Autodesk Inventor part; units mm, degrees
ref_plane "YZ Plane" through (0, 0, 0) normal (1, 0, 0) x (0, 1, 0)
ref_plane "XZ Plane" through (0, 0, 0) normal (0, 1, 0) x (-1, 0, 0)
ref_plane "XY Plane" through (0, 0, 0) normal (0, 0, 1) x (1, 0, 0)
sketch "Sketch1" plane through (0, 0, 0) normal (1, 0, 0) x (0, 1, 0)
  line L0 (109, 50) -> (-109, 50)
  line L1 (-109, 50) -> (-109, -50)
  line L2 (-109, -50) -> (109, -50)
  line L3 (109, -50) -> (109, 50)
  line L4 (109, 50) -> (-109, -50) construction
  line L5 (-109, 50) -> (109, -50) construction
  point P0 (0, 0)
  dimension "d0" = 100
  dimension "d1" = 218
extrude "Extrusion1" add sketch "Sketch1" along normal mid plane 10
sketch "Sketch2" plane through (-5, -109, 50) normal (0, 0, 1) x (1, 0, 0)
  line L0 (0, 218) -> (10, 218)
  line L1 (6, 218) -> (6, 196)
  line L2 (6, 196) -> (0, 190)
  line L3 (0, 218) -> (0, 0)
  line L4 (6, 218) -> (0, 218)
  line L5 (0, 190) -> (0, 218)
  line L6 (0, 0) -> (10, 0)
  line L7 (6, 0) -> (6, 60)
  line L8 (6, 60) -> (0, 60)
  line L9 (6, 0) -> (0, 0)
  line L10 (0, 60) -> (0, 0)
  point P0 (5, 109)
  dimension "d5" = 4
  dimension "d6" = 22
  dimension "d7" = 135
  dimension "d8" = 60
  dimension "d10" = 4
extrude "Extrusion2" cut sketch "Sketch2" against normal through all
sketch "Sketch3" plane through (5, 0, 0) normal (1, 0, 0) x (0, 0, -1)
  circle A0 centre (-38, -73) radius 4
  circle A1 centre (-23, -73) radius 4
  circle A2 centre (-8, -73) radius 4
  circle A3 centre (-33, 99) radius 4
  circle A4 centre (-18, 99) radius 4
  circle A5 centre (-3, 99) radius 4
  line L0 (-50, 109) -> (-50, -109)
  line L1 (-33, 99) -> (-18, 99) construction
  line L2 (-18, 99) -> (-3, 99) construction
  line L3 (50, 109) -> (-50, 109)
  line L4 (-38, -73) -> (-23, -73) construction
  line L5 (-23, -73) -> (-8, -73) construction
  line L6 (-50, -109) -> (50, -109)
  circle A6 centre (-20, 69) radius 5
  circle A7 centre (-5, 69) radius 5
  circle A8 centre (10, 69) radius 4
  circle A9 centre (-20, 9) radius 5
  circle A10 centre (-5, 9) radius 5
  circle A11 centre (10, 9) radius 4
  line L7 (-20, 69) -> (10, 69) construction
  line L8 (-20, 9) -> (10, 9) construction
  line L9 (-20, 9) -> (-20, 69) construction
  point P0 (0, 0)
  dimension "d13" = 8
  dimension "d14" = 8
  dimension "d15" = 17
  dimension "d16" = 15
  dimension "d17" = 15
  dimension "d18" = 10
  dimension "d19" = 12
  dimension "d20" = 15
  dimension "d21" = 15
  dimension "d22" = 36
  dimension "d23" = 10
  dimension "d24" = 8
  dimension "d25" = 40
  dimension "d26" = 30
  dimension "d27" = 15
  dimension "d28" = 15
  dimension "d29" = 60
  dimension "d30" = 15
  dimension "d31" = 15
extrude "Extrusion3" cut sketch "Sketch3" against normal through all
properties part number "DrivenSideBallScrewSupport"
Geometry: final body of the model. Coordinates: model frame, mm. A direction names the side the tool comes from. Coordinates: 2 decimals unless noted, no trailing zeros. Order: outer loops, then holes, each group sorted by start corner. A loop starts at its lowest first (then second) coordinate and runs counter-clockwise, first axis right, second up.
(1) Draft query along Y for faces 4 (the face through (3, 109, -1)), 5 (the face through (1, -2, -50)), 6 (the face through (0.07, 13.957, 5.651)), 7 (the face through (-2, -49, 1)). Return one class per face: pulls with the +Y half, pulls with the -Y half, needs draft (parallel to the pull), parting line crosses it, or undercut.
(2) Section query D-D (z = -42.5). Return the cut outline in (x, y), plus the area to 3 significant figures.
(3) Section query A-A (x = -2.25). Return the cut outline in (y, z).
(4) Section query B-B (z = -10). Return the cut outline in (x, y), plus the area to 3 significant figures.
(5) Access query for faces 1 (the face through (0.07, 65.095, -9.133)), 2 (the face through (1, 93, 1)), 3 (the face through (1, -79, 1)). Directions: +Z, -Z, +X, -X, +Y, -Y. A direction counts if a zero-diameter tool reaches every point of the face in a straight line with its end or side. Return the directions, or none.
(6) Section query C-C (y = -73). Return the cut outline in (x, z), plus the area to 3 significant figures.
(7) Material intervals for probe 1 along Y at (x, z) = (2.15, 23); probe 2 along Y at (x, z) = (-0.5, 5); probe 3 along Y at (x, z) = (2.5, 18), sorted ascending.
(8) First-contact query: pin 1 (11 mm diameter, centred on y = 101.5, z = 18, fed in from -X). Flat tip, straight axial feed; report the tip coordinate or a pass-through.
Solution:
1. face 4: pulls with the +Y half
1. face 5: needs draft
1. face 6: undercut
1. face 7: pulls with the -Y half
2. outline: (-5, -49) - (1, -49) - (1, -109) - (5, -109) - (5, 109) - (1, 109) - (1, 87) - (-5, 81) - close
2. area: 1,670 mm2
3. outline: (-49, -50) - (83.75, -50) - (83.75, 50) - (-49, 50) - close; hole circle Ø10 at (9, 5); hole circle Ø10 at (9, 20); hole circle Ø8 at (9, -10); hole circle Ø10 at (69, 5); hole circle Ø10 at (69, 20); hole circle Ø8 at (69, -10)
4. outline: (-5, -49) - (1, -49) - (1, -109) - (5, -109) - (5, 5) - (-5, 5) - close; (-5, 13) - (5, 13) - (5, 65) - (-5, 65) - close; (-5, 73) - (5, 73) - (5, 109) - (1, 109) - (1, 87) - (-5, 81) - close
4. area: 1,510 mm2
5. face 1: +X, -X
5. face 2: +Z, -Z, -X, +Y
5. face 3: +Z, -Z, -X, -Y
6. outline: (1, -50) - (5, -50) - (5, 4) - (1, 4) - close; (1, 12) - (5, 12) - (5, 19) - (1, 19) - close; (1, 27) - (5, 27) - (5, 34) - (1, 34) - close; (1, 42) - (5, 42) - (5, 50) - (1, 50) - close
6. area: 304 mm2
7. probe 1: y = -109 to -77, -69 to 5, 13 to 65, 73 to 109
7. probe 2: y = -49 to 4, 14 to 64, 74 to 85.5
7. probe 3: y = -109 to 4.42, 13.58 to 64.42, 73.58 to 95, 103 to 109
8. pin 1: stops at x = 1
